Design review of the part shown in the three views and the two pictorial views. Dimensions are in mm from the part's minimum x, y and z. Round coordinates to 2 decimals unless told otherwise and drop trailing zeros. Order: outer loops, then holes, each group sorted by start corner. A loop starts at its lowest first (then second) coordinate and runs counter-clockwise, first axis right, second up. Notation, with made-up numbers: (-25, -39.5) - (-11, -39.5) arc R26 ccw to (-11, -24.5) - close; hole circle Ø3 at (-3.75, 35.25). An arc over 180 degrees is marked (long way). One line per question, with ' | ' between items. Start each with the question number.
Item 1: Draft analysis for pull direction X (two halves, no side actions). For the marked faces 1 and 2, state which applies: +X half, -X half, draft (parallel to the pull), parting line (faces both ways), or undercut.
Item 2: Add section B-B on x = 48. State the section outline as (y, z) points.
Item 3: Insertion check: pin 1 Ø1 at (y, z) = (1, 6.5) entering from +X; pin 2 Ø1 at (y, z) = (3.5, 38.5) entering from +X; pin 3 Ø1 at (y, z) = (2, 44) entering from +X. Each pin has a flat end and moves straight along its axis. Give the tip position at first contact, or say it passes through.
Item 4: For L1, parallel to Z at x = 29, y = 1.4; L2, parallel to Z at x = 28, y = 2.1; L3, parallel to X at y = 1.75, z = 30, list the stretches that pass through material, from the lowest coordinate up. Write a range as [from, to].
Item 5: Add section D-D on x = 28.5. State how many separate pieces and enclosed holes the cut face has, and give its area (3 significant figures).
Item 6: Add section A-A on z = 30. State the section outline as (x, y) points.
Item 7: Add section C-C on z = 53. State the section outline as (x, y) points, and give its area (3 significant figures).
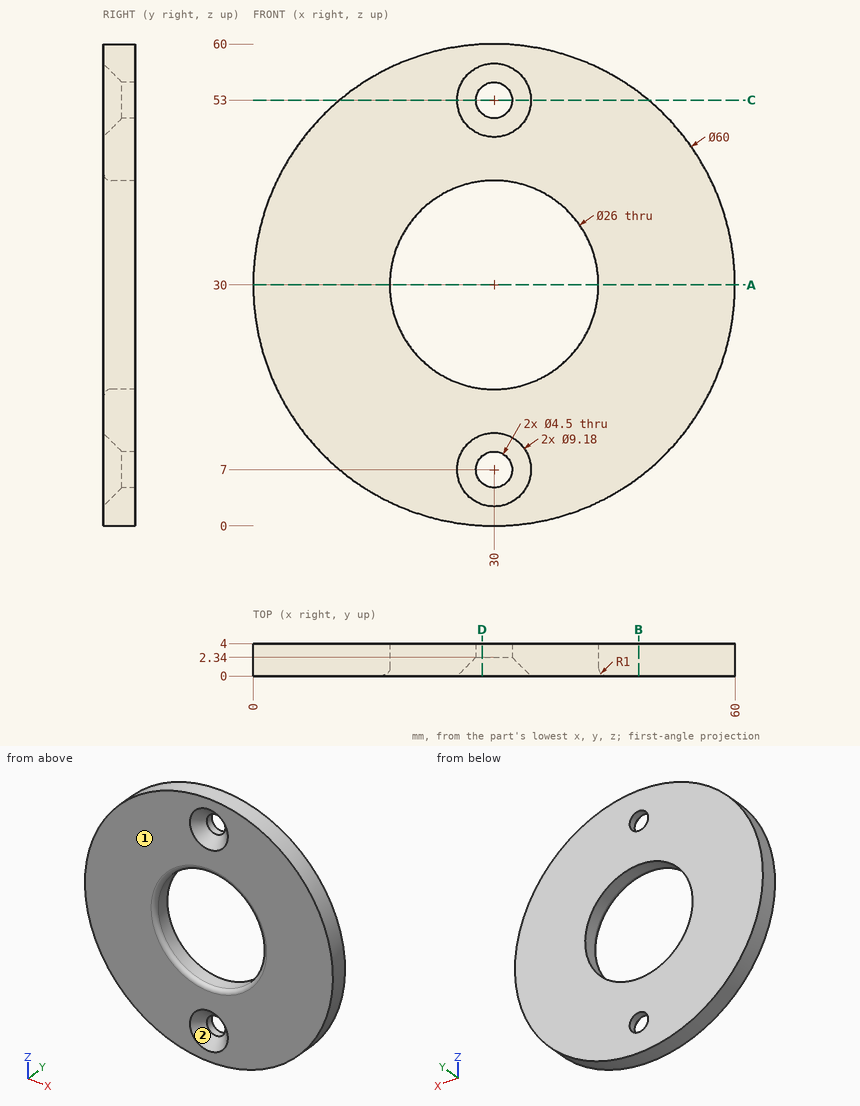
Determined:
1) face 1: draft | face 2: undercut
2) outline: (0, 6) - (4, 6) - (4, 54) - (0, 54) - close
3) pin 1: x = 49.26 | pin 2: x = 58.91 | pin 3: x = 56.79
4) L1: [0.02, 3.97], [10.03, 17.04], [42.96, 49.97], [56.03, 59.98] | L2: [0.07, 5.52], [8.48, 17.15], [42.85, 51.52], [54.48, 59.93] | L3: [0, 17], [43, 60]
5) separate pieces: 4 | enclosed holes: 0 | area: 96.2 mm2
6) outline: (0, 0) - (16, 0) arc R1 ccw to (17, 1) - (17, 4) - (0, 4) - close; (43, 1) arc R1 ccw to (44, 0) - (60, 0) - (60, 4) - (43, 4) - close
7) outline: (10.74, 0) - (25.41, 0) - (27.75, 2.34) - (27.75, 4) - (10.74, 4) - close; (32.25, 2.34) - (34.59, 0) - (49.26, 0) - (49.26, 4) - (32.25, 4) - close | area: 131 mm2
